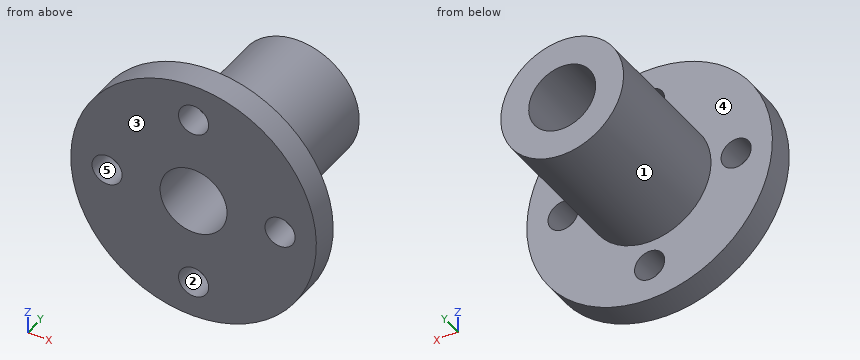
from build123d import *

# Parameters (mm, degrees)
SKETCH2_R          = 2.7
CUT_EXTRUDE1_DEPTH = 10


with BuildPart() as part:
    # Sketch1 → Revolve1 (revolve)
    with BuildSketch(Plane.XY, mode=Mode.PRIVATE) as revolve1_sk:
        Polygon((6, 0), (22, 0), (22, 5), (11, 5), (11, 31), (6, 31), align=None)
    revolve(revolve1_sk.sketch.rotate(Axis((0, 0, 0), (0, 1, 0)), 90), axis=Axis((0, 0, 0), (0, 1, 0)))  # turned: the seam where the file's is

    # Sketch2 → Cut-Extrude1 (cut)
    with BuildSketch(Plane.XZ):
        with Locations(Location((0, 15.5, 0), (0, 0, 270))):  # turned: the seam where the file's is
            Circle(SKETCH2_R)
        with Locations(Location((15.5, 0, 0), (0, 0, 270))):  # turned: the seam where the file's is
            Circle(SKETCH2_R)
        with Locations(Location((0, -15.5, 0), (0, 0, 270))):  # turned: the seam where the file's is
            Circle(SKETCH2_R)
        with Locations(Location((-15.5, 0, 0), (0, 0, 270))):  # turned: the seam where the file's is
            Circle(SKETCH2_R)
    extrude(amount=-CUT_EXTRUDE1_DEPTH, mode=Mode.SUBTRACT)


solid = part.part
Verification items for the finished model (mm, model axes). Face numbers are marked on the shaded views. A direction names the side the tool comes from. Coordinates: 2 decimals unless noted, no trailing zeros. Order: outer loops, then holes, each group sorted by start corner. A loop starts at its lowest first (then second) coordinate and runs counter-clockwise, first axis right, second up. Notation, with made-up numbers: (17.5, 36) -> (58.5, 36) arc R33 ccw to (58.5, 69) -> close; hole circle Ø6 at (13, 77). An arc over 180 degrees is marked (long way). Use CSV: the item, a comma, the result in double quotes. Start each with the question number.
Q1. Section check D-D, the plane z = 16. Record the cut outline in (x, y), and give its area (3 significant figures).
Q2. Section check B-B, the plane x = 14.5. Record the cut outline in (y, z).
Q3. Section check C-C, the plane x = 0. Record the cut outline in (y, z), and give its area (3 significant figures).
Q4. Section check A-A, the plane z = 0. Record the cut outline in (x, y), and give its area (3 significant figures).
Q5. Depth check by flat-ended pin: P1, Ø7, axis at x = 15.5, z = 0, coming from the +Y side; P2, Ø5, axis at x = -15.5, z = 0, coming from the -Y side; P3, Ø19, axis at x = 0, z = 0, coming from the +Y side; P4, Ø4, axis at y = 20.5, z = -10, coming from the -X side. Enter the tip coordinate at first touch or a pass-through.
Q6. Thickness scan on line 1 along X through (y, z) = (2.25, 0); line 2 along Y through (x, z) = (-10.5, 15); line 3 along Z through (x, y) = (5, 13.5). Record the ranges inside material, lowest first.
Q7. Tool access check on the marked faces 4 and 5. Record the directions out of +Z, -Z, +X, -X, +Y, -Y that give a thin tool (end or side, any length) a straight path to the whole face; none if there is none.
Q8. Draft check along Z on the marked faces 1, 2 and 3. Enter one of: +Z half, -Z half, draft (parallel to the pull), parting line (faces both ways), or undercut.
Returned:
1,outline,"(-15.1, 0) -> (-2.65, 0) -> (-2.65, 5) -> (-15.1, 5) -> close; (2.65, 0) -> (15.1, 0) -> (15.1, 5) -> (2.65, 5) -> close"
1,area,"124 mm^2"
2,outline,"(0, -16.55) -> (5, -16.55) -> (5, -2.51) -> (0, -2.51) -> close; (0, 2.51) -> (5, 2.51) -> (5, 16.55) -> (0, 16.55) -> close"
3,outline,"(0, -22) -> (5, -22) -> (5, -18.2) -> (0, -18.2) -> close; (0, -12.8) -> (5, -12.8) -> (5, -11) -> (31, -11) -> (31, -6) -> (0, -6) -> close; (0, 6) -> (31, 6) -> (31, 11) -> (5, 11) -> (5, 12.8) -> (0, 12.8) -> close; (0, 18.2) -> (5, 18.2) -> (5, 22) -> (0, 22) -> close"
3,area,"366 mm^2"
4,outline,"(-22, 0) -> (-18.2, 0) -> (-18.2, 5) -> (-22, 5) -> close; (-12.8, 0) -> (-6, 0) -> (-6, 31) -> (-11, 31) -> (-11, 5) -> (-12.8, 5) -> close; (6, 0) -> (12.8, 0) -> (12.8, 5) -> (11, 5) -> (11, 31) -> (6, 31) -> close; (18.2, 0) -> (22, 0) -> (22, 5) -> (18.2, 5) -> close"
4,area,"366 mm^2"
5,P1,"stops at y = 5"
5,P2,"passes through"
5,P3,"stops at y = 31"
5,P4,"stops at x = -7.55"
6,line 1,"x = -22 to -18.2, -12.8 to -6, 6 to 12.8, 18.2 to 22"
6,line 2,"y = 0 to 5"
6,line 3,"z = -9.8 to -3.32, 3.32 to 9.8"
7,face 4,"+Y"
7,face 5,"+Y, -Y"
8,face 1,"parting line"
8,face 2,"undercut"
8,face 3,"draft"
